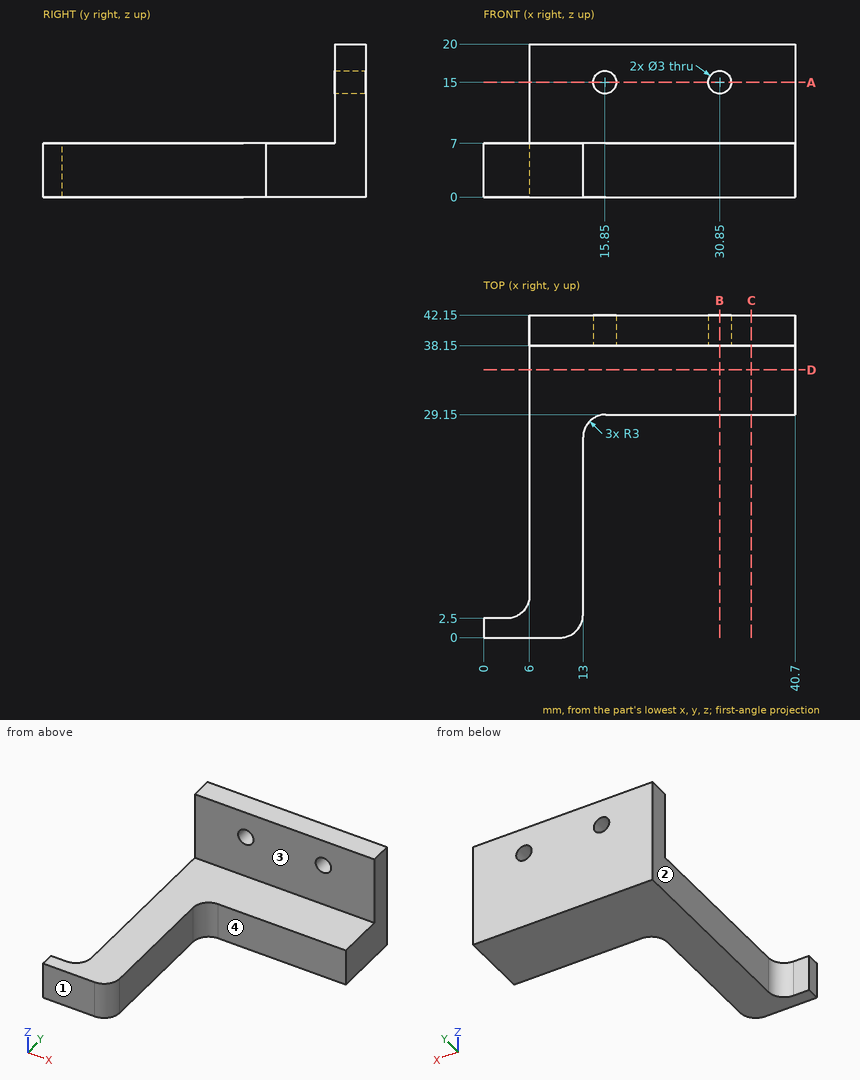
The figure shows three views and two pictorial views of one solid part (mm, origin at its lowest corner). Answer the questions. A direction names the side the tool comes from. Coordinates: 2 decimals unless noted, no trailing zeros. Loops run counter-clockwise (first coordinate to the right, second up) from the corner with the lowest first, then second, coordinate; pieces in that order, holes last. Notation, with made-up numbers: (43.25, -30) -> (48.25, -30) arc R9 cw to (48.25, -22) -> close; hole circle Ø2 at (-32, 47). An arc over 180 degrees is marked (long way). Use one line per item in the form item = value. Start each with the question number.
Item 1: A tool of negligible diameter and unlimited length cuts with its end or side. For the marked faces 1, 2, 3 and 4, from which of +Z, -Z, +X, -X, +Y, -Y can it reach the whole face along a straight path? Write none if from no direction.
Item 2: The part is cut by section D-D on y = 35. Determine the outline of the cut face in (x, z), then the cut area to 3 significant figures.
Item 3: Flat-ended cylindrical pins translate along their axes: pin 1 Ø4 at (x, z) = (15.85, 15) entering from -Y; pin 2 Ø1.5 at (x, z) = (2, 5) entering from +Y; pin 3 Ø10 at (y, z) = (23, 10.5) entering from -X; pin 4 Ø6 at (x, y) = (33, 24) entering from -Z. Find the tip coordinate at first contact, or state that the pin passes through.
Item 4: The part is cut by section A-A on z = 15. Determine the outline of the cut face in (x, y).
Item 5: The part is cut by section C-C on x = 35. Determine the outline of the cut face in (y, z).
Item 6: The part is cut by section B-B on x = 30.85. Determine the outline of the cut face in (y, z), then the cut area to 3 significant figures.
Item 7: Consider L1, parallel to X at y = 39.45, z = 15; L2, parallel to Y at x = 36, z = 6.25; L3, parallel to X at y = 11, z = 2.25. Determine where each line is inside the solid, lowest interval first. Write a range as [from, to].
Answer key:
q1.face_1 = +Z, -Z, +X, -X, -Y
q1.face_2 = +Z, -Z, -X, +Y
q1.face_3 = +Z, +X, -X, -Y
q1.face_4 = +Z, -Z, +X, -Y
q2.outline = (6, 0) -> (40.7, 0) -> (40.7, 7) -> (6, 7) -> close
q2.area = 243 mm2
q3.pin_1 = 38.15
q3.pin_2 = 2.5
q3.pin_3 = 6
q3.pin_4 = through
q4.outline = (6, 38.15) -> (14.35, 38.15) -> (14.35, 42.15) -> (6, 42.15) -> close; (17.35, 38.15) -> (29.35, 38.15) -> (29.35, 42.15) -> (17.35, 42.15) -> close; (32.35, 38.15) -> (40.7, 38.15) -> (40.7, 42.15) -> (32.35, 42.15) -> close
q5.outline = (29.15, 0) -> (42.15, 0) -> (42.15, 20) -> (38.15, 20) -> (38.15, 7) -> (29.15, 7) -> close
q6.outline = (29.15, 0) -> (42.15, 0) -> (42.15, 13.5) -> (38.15, 13.5) -> (38.15, 7) -> (29.15, 7) -> close; (38.15, 16.5) -> (42.15, 16.5) -> (42.15, 20) -> (38.15, 20) -> close
q6.area = 131 mm2
q7.L1 = [6, 14.35], [17.35, 29.35], [32.35, 40.7]
q7.L2 = [29.15, 42.15]
q7.L3 = [6, 13]
